The model under review builds one solid part; all positions refer to its coordinate system, in mm. Face numbers are marked on the shaded views. Give positions to 0.01 mm unless a question says otherwise; leave off trailing zeros. Order: outer loops, then holes, each group sorted by start corner. A loop starts at its lowest first (then second) coordinate and runs counter-clockwise, first axis right, second up.
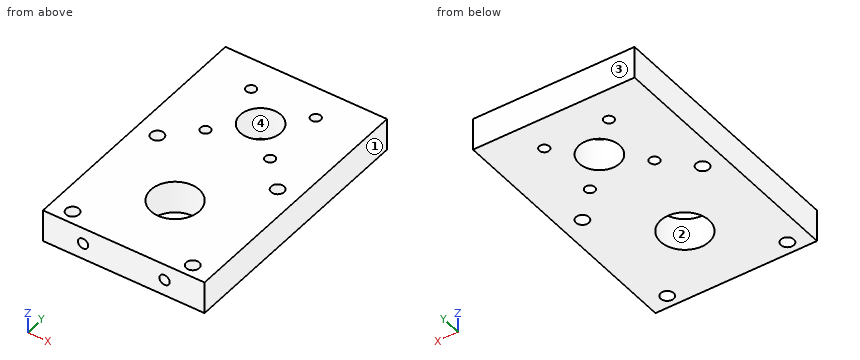
Autodesk Inventor part; units mm, degrees
ref_plane "YZ Plane" through (0, 0, 0) normal (1, 0, 0) x (0, 1, 0)
ref_plane "XZ Plane" through (0, 0, 0) normal (0, 1, 0) x (-1, 0, 0)
ref_plane "XY Plane" through (0, 0, 0) normal (0, 0, 1) x (1, 0, 0)
sketch "Sketch1" plane through (0, 0, 0) normal (0, 0, 1) x (1, 0, 0)
  line L0 (0, 0.3892) -> (63.5, 0.3892)
  line L1 (63.5, 0.3892) -> (63.5, 101.9892)
  line L2 (63.5, 101.9892) -> (0, 101.9892)
  line L3 (0, 101.9892) -> (0, 0.3892)
  point P0 (0, 0)
  dimension "d0" = 63.5
  dimension "d1" = 101.6
extrude "Extrusion1" add sketch "Sketch1" along normal blind 12.7
hole "Hole15" at (8.128, 5.3422, 12.7) direction (0, 0, -1) diameter 5.08 end through all
hole "Hole16" at (55.372, 5.3422, 12.7) direction (0, 0, -1) diameter 5.08 end through all
hole "Hole17" at (8.128, 52.5862, 12.7) direction (0, 0, -1) diameter 5.08 end through all
hole "Hole18" at (55.372, 52.5862, 12.7) direction (0, 0, -1) diameter 5.08 end through all
hole "Hole19" at (31.75, 76.5892, 12.7) direction (0, 0, -1) diameter 15.9766 end through all
hole "Hole20" at (31.75, 28.9642, 12.7) direction (0, 0, -1) diameter 19.05 end through all
hole "Hole23" at (15.748, 0.3892, 6.35) direction (0, 1, 0) diameter 4.0386 depth 50.8 tip angle 118
hole "Hole24" at (47.752, 0.3892, 6.35) direction (0, 1, 0) diameter 4.0386 depth 50.8 tip angle 118
sketch "Font" plane through (0, 0, 12.7) normal (0, 0, 1) x (1, 0, 0)
  circle A0 centre (31.75, 28.9642) radius 9.525
  circle A1 centre (31.75, 76.5892) radius 7.9883
  circle A2 centre (55.372, 52.5862) radius 2.54
  circle A3 centre (8.128, 52.5862) radius 2.54
  circle A4 centre (55.372, 5.3422) radius 2.54
  circle A5 centre (8.128, 5.3422) radius 2.54
  line L0 (0, 0.3892) -> (0, 101.9892)
  line L1 (63.5, 0.3892) -> (0, 0.3892)
  line L2 (63.5, 101.9892) -> (63.5, 0.3892)
  line L3 (0, 101.9892) -> (63.5, 101.9892)
  point P0 (0, 0)
  dimension "d220" = 101.6
  dimension "d221" = 5.08
  dimension "d222" = 15.9766
  dimension "d223" = 19.05
  dimension "d224" = 8.128
  dimension "d225" = 4.953
  dimension "d226" = 28.575
  dimension "d227" = 76.2
  dimension "d228" = 8.128
  dimension "d229" = 4.953
  dimension "d230" = 52.197
  dimension "d231" = 52.197
  dimension "d237" = 31.75
  dimension "d238" = 31.75
sketch "Side" plane through (0, 0.3892, 0) normal (0, -1, 0) x (1, 0, 0)
  circle A0 centre (47.752, 6.35) radius 2.0193
  circle A1 centre (15.748, 6.35) radius 2.0193
  line L0 (63.5, 12.7) -> (0, 12.7)
  line L1 (0, 0) -> (0, 12.7)
  line L2 (0, 0) -> (63.5, 0)
  line L3 (63.5, 0) -> (63.5, 12.7)
  dimension "d232" = 15.748
  dimension "d233" = 12.7
  dimension "d234" = 15.748
  dimension "d235" = 6.35
  dimension "d236" = 6.35
hole "Hole25" at (19.05, 89.2892, 12.7) direction (0, 0, -1) diameter 3.937 end through all
hole "Hole26" at (19.05, 63.8892, 12.7) direction (0, 0, -1) diameter 3.937 end through all
hole "Hole27" at (44.45, 89.2892, 12.7) direction (0, 0, -1) diameter 3.937 end through all
hole "Hole28" at (44.45, 63.8892, 12.7) direction (0, 0, -1) diameter 3.937 end through all
sketch "Sketch5" plane through (0, 0, 12.7) normal (0, 0, 1) x (1, 0, 0)
  circle A0 centre (44.45, 63.8892) radius 1.9685
  circle A1 centre (44.45, 89.2892) radius 1.9685
  circle A2 centre (19.05, 63.8892) radius 1.9685
  circle A3 centre (19.05, 89.2892) radius 1.9685
  circle A4 centre (31.75, 28.9642) radius 9.525
  circle A5 centre (31.75, 76.5892) radius 7.9883
  circle A6 centre (55.372, 52.5862) radius 2.54
  circle A7 centre (8.128, 52.5862) radius 2.54
  circle A8 centre (55.372, 5.3422) radius 2.54
  circle A9 centre (8.128, 5.3422) radius 2.54
  line L0 (0, 0.3892) -> (0, 101.9892)
  line L1 (63.5, 0.3892) -> (0, 0.3892)
  line L2 (63.5, 101.9892) -> (63.5, 0.3892)
  line L3 (0, 101.9892) -> (63.5, 101.9892)
  point P0 (0, 0)
  dimension "d275" = 63.5
  dimension "d276" = 19.05
  dimension "d277" = 44.45
  dimension "d278" = 88.9
properties part number "ytowerv1"
Item 1: Take a section at C-C (z = 10.5). Give the number of separate pieces and of enclosed holes in the cut face, and give its area (3 significant figures).
Values found:
separate pieces: 1
enclosed holes: 10
area: 5,840 mm2
Item 2: Draft analysis for pull direction Y (two halves, no side actions). For the marked faces 1, 2, 3 and 4, state which applies: released by +Y, released by -Y, zero draft, split by the parting line, or undercut.
Values found:
face 1: zero draft
face 2: undercut
face 3: released by +Y
face 4: undercut
Item 3: Take a section at D-D (y = 76.5). Give the boundary of the cut face in (x, z).
Values found:
outline: (0, 0) - (23.76, 0) - (23.76, 12.7) - (0, 12.7) - close; (39.74, 0) - (63.5, 0) - (63.5, 12.7) - (39.74, 12.7) - close
Item 4: Take a section at B-B (y = 21). Give the boundary of the cut face in (x, z).
Values found:
outline: (0, 0) - (26.53, 0) - (26.53, 12.7) - (0, 12.7) - close; (36.97, 0) - (63.5, 0) - (63.5, 12.7) - (36.97, 12.7) - close; hole circle Ø4.04 at (15.75, 6.35); hole circle Ø4.04 at (47.75, 6.35)
Item 5: Clearance check with a flat-ended pin moving along its axis: pin 1 Ø22 at (x, y) = (31.75, 28.96) entering from -Z. State where the tip first meets the part, or that it passes through.
Values found:
pin 1: stops at z = 0
Item 6: Take a section at A-A (x = 19.05). Give the boundary of the cut face in (y, z), and give its area (3 significant figures).
Values found:
outline: (0.39, 0) - (61.92, 0) - (61.92, 12.7) - (0.39, 12.7) - close; (65.86, 0) - (87.32, 0) - (87.32, 12.7) - (65.86, 12.7) - close; (91.26, 0) - (101.99, 0) - (101.99, 12.7) - (91.26, 12.7) - close
area: 1,190 mm2
Item 7: For line 1 (Y direction, x = 31.75, z = 8.5); line 2 (Y direction, x = 44.45, z = 4); line 3 (X direction, y = 17, z = 6.35), list the stretches that pass through material, from the lowest coordinate up.
Values found:
line 1: y = 0.39 to 19.44, 38.49 to 68.6, 84.58 to 101.99
line 2: y = 0.39 to 61.92, 65.86 to 87.32, 91.26 to 101.99
line 3: x = 0 to 13.73, 17.77 to 45.73, 49.77 to 63.5
